from build123d import *

# Parameters (mm, degrees)
F1_DEPTH = 65
F2_R     = 5
F3_DEPTH = 25
F5_DEPTH = 25
F6_R     = 1
F8_DEPTH = 15


with BuildPart() as f1:
    # F0 (on Top) → F1 (new body)
    with BuildSketch(Plane.XY):
        with BuildLine():
            Line((30.1594209448, 52.9782638401), (12.1594209448, 52.9782638401))
            Line((12.1594209448, 52.9782638401), (12.1594209448, 48.9782638401))
            Line((12.1594209448, 48.9782638401), (30.1594209448, 48.9782638401))
            ThreePointArc((30.1594209448, 48.9782638401), (34.4020616319, 47.2209045272), (36.1594209448, 42.9782638401))
            Line((36.1594209448, 42.9782638401), (36.1594209448, 7.9782638401))
            ThreePointArc((36.1594209448, 7.9782638401), (34.4020616319, 3.735623153), (30.1594209448, 1.9782638401))
            Line((30.1594209448, 1.9782638401), (-59.8505790552, 1.9782638401))
            Line((-59.8505790552, 1.9782638401), (-59.8505790552, -2.0217361599))
            Line((-59.8505790552, -2.0217361599), (30.1594209448, -2.0217361599))
            ThreePointArc((30.1594209448, -2.0217361599), (37.2304887566, 0.9071960282), (40.1594209448, 7.9782638401))
            Line((40.1594209448, 7.9782638401), (40.1594209448, 42.9782638401))
            ThreePointArc((40.1594209448, 42.9782638401), (37.2304887566, 50.0493316519), (30.1594209448, 52.9782638401))
        make_face()
    extrude(amount=F1_DEPTH)

    # F2 (on face) → F3 (cut)
    with BuildSketch(Plane(origin=(0, 52.9782638401, 0), x_dir=(-1, 0, 0), z_dir=(0, 1, 0))):
        with Locations((-21.1594209448, 10)):
            Circle(F2_R)
        with Locations((-21.1594209448, 55)):
            Circle(F2_R)
    extrude(amount=-F3_DEPTH, mode=Mode.SUBTRACT)

    # F4 (on face) → F5 (cut)
    with BuildSketch(Plane.XZ.offset(2.0217361599)):
        with BuildLine():
            Line((-59.8505790552, 65), (-59.8505790552, 0))
            ThreePointArc((-59.8505790552, 0), (-35.838071233, 32.5), (-59.8505790552, 65))
        make_face()
    extrude(amount=-F5_DEPTH, mode=Mode.SUBTRACT)

    # F6
    f6_edges = [f1.edges().sort_by_distance(p)[0] for p in [
        (-59.850579, -0.021736, 65),
        (-59.850579, -0.021736, 0),
    ]]
    fillet(f6_edges, radius=F6_R)

    # F7 (on face) → F8 (cut)
    with BuildSketch(Plane.XZ.offset(2.0217361599)):
        with BuildLine():
            ThreePointArc((14.6594209448, 27), (20.1594209448, 32.5), (14.6594209448, 38))
            Line((14.6594209448, 38), (5.6594209448, 38))
            ThreePointArc((5.6594209448, 38), (0, 32.5), (5.6594209448, 27))
            Line((5.6594209448, 27), (10.1594209448, 27))
            Line((10.1594209448, 27), (14.6594209448, 27))
        make_face()
    extrude(amount=-F8_DEPTH, mode=Mode.SUBTRACT)


solid = f1.part
For this review, take the finished solid that the model builds, in its own axes (mm). A direction names the side the tool comes from. Coordinates: 2 decimals unless noted, no trailing zeros. Loops run counter-clockwise (first coordinate to the right, second up) from the corner with the lowest first, then second, coordinate; pieces in that order, holes last. Notation, with made-up numbers: (-17.5, 23.25) - (-0.5, 23.25) arc R23 cw to (-0.5, 43.25) - close; hole circle Ø9 at (46, 36.25). An arc over 180 degrees is marked (long way). Return JSON: item names as keys, results as strings.
Item 1: Take a section at A-A (z = 32.5). Give the boundary of the cut face in (x, y), then the cut area to 3 significant figures.
Determined:
{"outline": "(-35.84, -2.02) - (0, -2.02) - (0, 1.98) - (-35.84, 1.98) - close; (12.16, 48.98) - (30.16, 48.98) arc R6 cw to (36.16, 42.98) - (36.16, 7.98) arc R6 cw to (30.16, 1.98) - (20.16, 1.98) - (20.16, -2.02) - (30.16, -2.02) arc R10 ccw to (40.16, 7.98) - (40.16, 42.98) arc R10 ccw to (30.16, 52.98) - (12.16, 52.98) - close", "area": "496 mm2"}
Item 2: For faces 1 (the flat face through (12.159, 51, 32)), 2 (the cylindrical face through (16.39, 51.01, 11.5)), 3 (the flat face through (36.159, 26, 32)), 4 (the cylindrical face through (0, 0, 32.6)), list the 3-axis set-ups (+Z, -Z, +X, -X, +Y, -Y) from which the entire face can be reached by the end or side of a thin tool; tool diameter is ignored.
Determined:
{"face 1": "+Z, -Z, -X, +Y", "face 2": "+Y", "face 3": "+Z, -Z, -X", "face 4": "+Y, -Y"}
Item 3: Insertion check: pin 1 (2 mm diameter, centred on x = -3, z = 31.5, fed in from +Y); pin 2 (2 mm diameter, centred on x = 10, y = 0, fed in from -Z); pin 3 (1.5 mm diameter, centred on y = 17, z = 11, fed in from -X); pin 4 (3 mm diameter, centred on y = 52, z = 23, fed in from -X). Each pin has a flat end and moves straight along its axis. Give the tip position at first contact, or say it passes through.
Determined:
{"pin 1": "stops at y = 1.98", "pin 2": "stops at z = 0", "pin 3": "stops at x = 36.16", "pin 4": "stops at x = 12.16"}
Item 4: For line 1 (Y direction, x = 30.5, z = 60.5); line 2 (Y direction, x = 13.5, z = 32.5); line 3 (Y direction, x = -11, z = 22), list the stretches that pass through material, from the lowest coordinate up.
Determined:
{"line 1": "y = -2.02 to 1.99, 48.97 to 52.97", "line 2": "y = 48.98 to 52.98", "line 3": "y = -2.02 to 1.98"}
Item 5: Take a section at C-C (x = -37). Give the boundary of the cut face in (y, z), then the cut area to 4 significant figures.
Determined:
{"outline": "(-2.02, 0) - (1.98, 0) - (1.98, 23.69) - (-2.02, 23.69) - close; (-2.02, 41.31) - (1.98, 41.31) - (1.98, 65) - (-2.02, 65) - close", "area": "189.5 mm2"}
Item 6: Take a section at B-B (x = 24.5). Give the boundary of the cut face in (y, z).
Determined:
{"outline": "(-2.02, 0) - (1.98, 0) - (1.98, 65) - (-2.02, 65) - close; (48.98, 0) - (52.98, 0) - (52.98, 6.28) - (48.98, 6.28) - close; (48.98, 13.72) - (52.98, 13.72) - (52.98, 51.28) - (48.98, 51.28) - close; (48.98, 58.72) - (52.98, 58.72) - (52.98, 65) - (48.98, 65) - close"}
Item 7: Take a section at D-D (y = 10.5). Give the boundary of the cut face in (x, z), then the cut area to 3 significant figures.
Determined:
{"outline": "(36.16, 0) - (40.16, 0) - (40.16, 65) - (36.16, 65) - close", "area": "260 mm2"}
Item 8: Mouldability with a two-part tool opening along Z and no side actions: class faces 5 (the flat face through (-3, 1.978, 32)), 6 (the flat face through (10, 1, 0)), 7 (the flat face through (10, 0, 27)) as pulls with the +Z half, pulls with the -Z half, needs draft (parallel to the pull), parting line crosses it, or undercut.
Determined:
{"face 5": "needs draft", "face 6": "pulls with the -Z half", "face 7": "undercut"}
